Design review of the part built by this model. Coordinates are the model's own, in mm. A direction names the side the tool comes from. Round coordinates to 2 decimals unless told otherwise and drop trailing zeros. Loops run counter-clockwise (first coordinate to the right, second up) from the corner with the lowest first, then second, coordinate; pieces in that order, holes last. Notation, with made-up numbers: (79, 55.5) - (99, 55.5) arc R26 ccw to (99, 72.5) - close; hole circle Ø9 at (3.25, 68). An arc over 180 degrees is marked (long way). Answer as CSV lines item,"result". Start each with the question number.
(1) Wall thickness on L1, parallel to X at y = -3, z = -60; L2, parallel to Y at x = 15, z = -54.5: over which ranges is each line inside the solid? List them lowest first.
(2) Consider section A-A (y = -2). Give the boundary of the cut face in (x, z).
(3) Consider section C-C (y = 16). Give the boundary of the cut face in (x, z), and give its area (3 significant figures).
(4) Mouldability with a two-part tool opening along X and no side actions: class faces 1 (the flat face through (3, 0, -64.5)), 2 (the flat face through (-20.95, -24, 1)), 3 (the cylindrical face through (-8.71, 19.64, 2.42)), 4 (the flat face through (13.95, -6, 1)) as released by +X, released by -X, zero draft, split by the parting line, or undercut.
(5) Consider section D-D (y = -13.5). Give the boundary of the cut face in (x, z), and give its area (3 significant figures).
(6) For P1, Ø6, axis at y = 26.5, z = 24.5, coming from the -X side; P2, Ø1, axis at y = 1, z = 32.5, coming from the +X side; P3, Ø12, axis at x = -2, y = 3, coming from the +Z side, all flat-tipped, find the tip position at first contact; note any pin that passes through.
(7) Consider section B-B (z = 27.5). Give the boundary of the cut face in (x, y), and give its area (3 significant figures).
(8) For faces 5 (the flat face through (-13.95, -5, 1)), 6 (the flat face through (17, -22.05, 1)), 7 (the flat face through (12.2, 0, 2)), list the 3-axis set-ups (+Z, -Z, +X, -X, +Y, -Y) from which the entire face can be reached by the end or side of a thin tool; tool diameter is ignored.
from build123d import *

# Parameters (mm, degrees)
BOSS_EXTRUDE1_DEPTH = 67.5
BOSS_EXTRUDE2_START = -3
BOSS_EXTRUDE2_DEPTH = 3
SKETCH6_W           = 6
SKETCH6_H           = 6.75
BOSS_EXTRUDE3_DEPTH = 135
SKETCH7_W           = 1
SKETCH7_H           = 40.05
CUT_EXTRUDE2_DEPTH  = 140.881753635


with BuildPart() as part:
    # Sketch2 → Boss-Extrude1 (new, symmetric)
    with BuildSketch(Plane.XY):
        with BuildLine():
            Line((-13.95, 11.1), (-13.95, -11.1))
            Line((-13.95, -11.1), (-13.95, -22.05))
            Line((-13.95, -22.05), (-20.95, -22.05))
            Line((-20.95, -22.05), (-20.95, -25.05))
            Line((-20.95, -25.05), (20.95, -25.05))
            Line((20.95, -25.05), (20.95, -22.05))
            Line((20.95, -22.05), (13.95, -22.05))
            Line((13.95, -22.05), (13.95, -11.1))
            Line((13.95, -11.1), (13.95, 11.1))
            ThreePointArc((13.95, 11.1), (0, 25.05), (-13.95, 11.1))
        make_face()
        with BuildLine():
            Line((12.2, -11.1), (12.2, 11.1))
            ThreePointArc((12.2, 11.1), (0, 23.3), (-12.2, 11.1))
            Line((-12.2, 11.1), (-12.2, -11.1))
            ThreePointArc((-12.2, -11.1), (0, -23.3), (12.2, -11.1))
        make_face(mode=Mode.SUBTRACT)
    extrude(amount=BOSS_EXTRUDE1_DEPTH, both=True)

    # Sketch5 → Boss-Extrude2 (add)
    with BuildSketch(Plane(origin=(0, 0, -67.5), x_dir=(-1, 0, 0), z_dir=(0, 0, -1)).offset(BOSS_EXTRUDE2_START)):
        with BuildLine():
            Line((-13.95, 11.1), (-13.95, -22.05))
            Line((-13.95, -22.05), (-20.95, -22.05))
            Line((-20.95, -22.05), (-20.95, -25.05))
            Line((-20.95, -25.05), (20.95, -25.05))
            Line((20.95, -25.05), (20.95, -22.05))
            Line((20.95, -22.05), (13.95, -22.05))
            Line((13.95, -22.05), (13.95, 11.1))
            ThreePointArc((13.95, 11.1), (0, 25.05), (-13.95, 11.1))
        make_face()
    extrude(amount=BOSS_EXTRUDE2_DEPTH)

    # Sketch6 → Boss-Extrude3 (add)
    with BuildSketch(Plane.XY.offset(67.5)):
        with Locations((0, 26.675)):
            Rectangle(SKETCH6_W, SKETCH6_H)
    extrude(amount=-BOSS_EXTRUDE3_DEPTH)

    # Sketch7 → Cut-Extrude2 (cut, through all)
    with BuildSketch(Plane.XY.offset(67.5)):
        with Locations((0, 10.025)):
            Rectangle(SKETCH7_W, SKETCH7_H)
    extrude(amount=-CUT_EXTRUDE2_DEPTH, mode=Mode.SUBTRACT)


solid = part.part
Determined:
1,L1,"x = -13.95 to -12.2, 12.2 to 13.95"
1,L2,"y = -25.05 to -22.05"
2,outline,"(-13.95, -67.5) - (-0.5, -67.5) - (-0.5, -64.5) - (-12.2, -64.5) - (-12.2, 67.5) - (-13.95, 67.5) - close; (0.5, -67.5) - (13.95, -67.5) - (13.95, 67.5) - (12.2, 67.5) - (12.2, -64.5) - (0.5, -64.5) - close"
3,outline,"(-13.06, -67.5) - (-0.5, -67.5) - (-0.5, -64.5) - (-11.17, -64.5) - (-11.17, 67.5) - (-13.06, 67.5) - close; (0.5, -67.5) - (13.06, -67.5) - (13.06, 67.5) - (11.17, 67.5) - (11.17, -64.5) - (0.5, -64.5) - close"
3,area,"574 mm^2"
4,face 1,"undercut"
4,face 2,"released by -X"
4,face 3,"undercut"
4,face 4,"released by +X"
5,outline,"(-13.95, -67.5) - (13.95, -67.5) - (13.95, 67.5) - (11.96, 67.5) - (11.96, -64.5) - (-11.96, -64.5) - (-11.96, 67.5) - (-13.95, 67.5) - close"
5,area,"609 mm^2"
6,P1,"stops at x = -6.39"
6,P2,"stops at x = 13.95"
6,P3,"stops at z = -64.5"
7,outline,"(-20.95, -25.05) - (20.95, -25.05) - (20.95, -22.05) - (13.95, -22.05) - (13.95, 11.1) arc R13.95 ccw to (3, 24.72) - (3, 30.05) - (0.5, 30.05) - (0.5, 23.29) arc R12.2 cw to (12.2, 11.1) - (12.2, -11.1) arc R12.2 cw to (-12.2, -11.1) - (-12.2, 11.1) arc R12.2 cw to (-0.5, 23.29) - (-0.5, 30.05) - (-3, 30.05) - (-3, 24.72) arc R13.95 ccw to (-13.95, 11.1) - (-13.95, -22.05) - (-20.95, -22.05) - close"
7,area,"371 mm^2"
8,face 5,"+Z, -Z, -X, +Y"
8,face 6,"+Z, -Z, +X, +Y"
8,face 7,"+Z"
